from build123d import *

# Parameters (mm, degrees)
F0_W     = 292.1
F0_H     = 292.1
F1_DEPTH = 50.8
F2_T     = -3.571875
F3_R     = 5.08


with BuildPart() as f1:
    # F0 (on Top) → F1 (new body)
    with BuildSketch(Plane.XY):
        with Locations((-56.953185622, -2.171928063)):
            Rectangle(F0_W, F0_H)
    extrude(amount=F1_DEPTH)

    # F2
    f2_openings = [f1.faces().sort_by_distance(p)[0] for p in [
        (-56.953186, -148.221928, 25.4),
        (-56.953186, 143.878072, 25.4),
        (-56.953186, -2.171928, 0),
    ]]
    offset(amount=F2_T, openings=f2_openings)

    # F3
    f3_edges = [f1.edges().sort_by_distance(p)[0] for p in [
        (-199.431311, -2.171928, 47.228125),
        (85.524939, -2.171928, 47.228125),
        (-203.003186, -2.171928, 50.8),
        (89.096814, -2.171928, 50.8),
    ]]
    fillet(f3_edges, radius=F3_R)


solid = f1.part
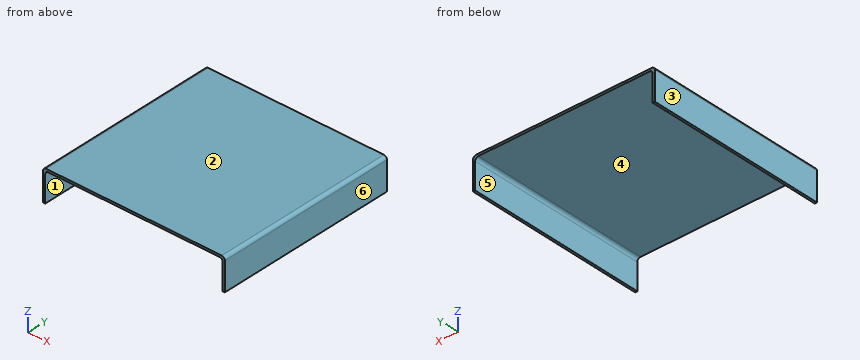
Can you work these out from the model? Positions are in its coordinate system, mm. Face numbers are marked on the shaded views. A direction names the side the tool comes from. Give positions to 0.01 mm unless a question says otherwise; leave off trailing zeros. Write each loop counter-clockwise with the first axis right and the second up, starting at its lowest first coordinate (ties: lowest second). Pieces come first, ordered by that corner, then holes. Notation, with made-up numbers: M 58.25,5.25 L 110.25,5.25 A22 cw 110.25,19.25 Z; hole C 67,60.5 d11. An arc over 180 degrees is marked long. Answer in a Markdown table with one row per item. Add a question column.
Item 1: Imagine slicing it at A-A, the plane z = 38. Write out the boundary of the cut face in (x, y).
Item 2: Please list where these lines run through material, in increasing order: L1, parallel to X at y = 52, z = 23.5; L2, parallel to Z at x = -99, y = 46.
Item 3: For pin 1 Ø5 at (x, y) = (-98.5, 82) entering from -Z; pin 2 Ø8 at (x, z) = (41, 44) entering from -Y, each with a flat end and sliding along its axis, tell me the tip position at first contact or that it passes through.
Item 4: Imagine slicing it at B-B, the plane y = 126.5. Write out the boundary of the cut face in (x, z).
Item 5: We'd pull the mould along X, two halves only. Please class the marked faces 1, 2, 3 and 4: released by +X, released by -X, zero draft, split by the parting line, or undercut.
Item 6: Imagine slicing it at C-C, the plane x = -108. Write out the boundary of the cut face in (y, z).
Item 7: On a 3-axis mill with a long thin cutter (end or side, diameter ignored), from which of +Z, -Z, +X, -X, +Y, -Y can I reach the whole of each face in a straight line? I mean the marked faces 5 and 6. Say none if no direction works.
Evaluation:
| question | item | result |
|---|---|---|
| 1 | outline | M -203,-148.22 L -199.43,-148.22 L -199.43,143.88 L -203,143.88 Z; M 85.52,-148.22 L 89.1,-148.22 L 89.1,143.88 L 85.52,143.88 Z |
| 2 | L1 | x = -203 to -199.43, 85.52 to 89.1 |
| 2 | L2 | z = 47.23 to 50.8 |
| 3 | pin 1 | stops at z = 47.23 |
| 3 | pin 2 | stops at y = -148.22 |
| 4 | outline | M -203,0 L -199.43,0 L -199.43,42.15 A5.08 cw -194.35,47.23 L 80.44,47.23 A5.08 cw 85.52,42.15 L 85.52,0 L 89.1,0 L 89.1,45.72 A5.08 ccw 84.02,50.8 L -197.92,50.8 A5.08 ccw -203,45.72 Z |
| 5 | face 1 | undercut |
| 5 | face 2 | zero draft |
| 5 | face 3 | released by -X |
| 5 | face 4 | undercut |
| 6 | outline | M -148.22,47.23 L 143.88,47.23 L 143.88,50.8 L -148.22,50.8 Z |
| 7 | face 5 | -Z, +Y, -Y |
| 7 | face 6 | +Z, -Z, +X, +Y, -Y |
